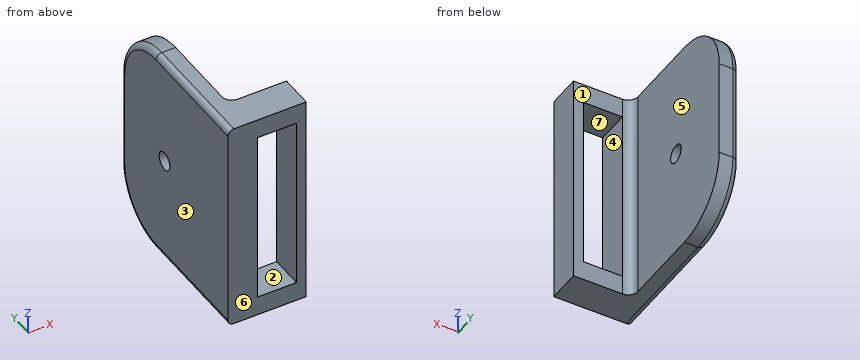
```python
from build123d import *

# Parameters (mm, degrees)
SKETCH1_W           = 40
SKETCH1_H           = 110
BOSS_EXTRUDE1_DEPTH = 17
SKETCH4_W           = 110
SKETCH4_H           = 75
BOSS_EXTRUDE2_DEPTH = 10
SKETCH5_W           = 20
SKETCH5_H           = 90
CUT_EXTRUDE1_DEPTH  = 17
SKETCH6_R           = 4.6
CUT_EXTRUDE2_DEPTH  = 10
FILLET1_R           = 30
FILLET2_R           = 3
FILLET3_R           = 5


with BuildPart() as part:
    # Sketch1 → Boss-Extrude1 (new body)
    with BuildSketch(Plane(origin=(0, 0, 0), x_dir=(1, 0, 0), z_dir=(0, 1, 0))):
        with Locations((20, 55)):
            Rectangle(SKETCH1_W, SKETCH1_H)
    extrude(amount=BOSS_EXTRUDE1_DEPTH)

    # Sketch4 → Boss-Extrude2 (add)
    with BuildSketch(Plane(origin=(0, 0, 0), x_dir=(0, 0, -1), z_dir=(1, 0, 0))):
        with Locations((55, 54.5)):
            Rectangle(SKETCH4_W, SKETCH4_H)
    extrude(amount=BOSS_EXTRUDE2_DEPTH)

    # Sketch5 → Cut-Extrude1 (cut)
    with BuildSketch(Plane(origin=(0, 17, 0), x_dir=(1, 0, 0), z_dir=(0, 1, 0))):
        with Locations((25, 55)):
            Rectangle(SKETCH5_W, SKETCH5_H)
    extrude(amount=-CUT_EXTRUDE1_DEPTH, mode=Mode.SUBTRACT)

    # Sketch6 → Cut-Extrude2 (cut)
    with BuildSketch(Plane(origin=(10, 0, 0), x_dir=(0, 0, -1), z_dir=(1, 0, 0))):
        with Locations((55, 54.7)):
            Circle(SKETCH6_R)
    extrude(amount=-CUT_EXTRUDE2_DEPTH, mode=Mode.SUBTRACT)

    # Fillet1
    fillet1_edges = [part.edges().sort_by_distance(p)[0] for p in [
        (5, 92, 0),
        (5, 92, -110),
    ]]
    fillet(fillet1_edges, radius=FILLET1_R)

    # Fillet2
    fillet2_edges = [part.edges().sort_by_distance(p)[0] for p in [
        (0, 31, 0),
        (0, 92, -55),
        (0, 31, -110),
        (0, 83.213203436, -101.213203436),
        (0, 83.213203436, -8.786796564),
    ]]
    fillet(fillet2_edges, radius=FILLET2_R)

    # Fillet3
    fillet3_edges = [part.edges().sort_by_distance(p)[0] for p in [
        (10, 17, -55),
    ]]
    fillet(fillet3_edges, radius=FILLET3_R - 0.0001)  # a hair under: the kernel refuses the full size


solid = part.part
```
Geometry: final body of the model. Coordinates: model frame, mm. Face numbers are marked on the shaded views. A direction names the side the tool comes from. Round coordinates to 2 decimals unless told otherwise and drop trailing zeros. Order: outer loops, then holes, each group sorted by start corner. A loop starts at its lowest first (then second) coordinate and runs counter-clockwise, first axis right, second up. Notation, with made-up numbers: (56.25, 27.25) -> (63.25, 27.25) arc R29 ccw to (63.25, 61.25) -> close; hole circle Ø11 at (-4, -24.75). An arc over 180 degrees is marked (long way). Use CSV: the item, a comma, the result in double quotes. Start each with the question number.
1) Section B-B (z = -55). State how many separate pieces and enclosed holes the cut face has, and give its area (3 significant figures).
2) First-contact query: pin 1 Ø4 at (y, z) = (41, -82.5) entering from +X; pin 2 Ø20 at (x, z) = (28, -42.5) entering from +Y. Flat tips, straight axial feed; report the tip coordinate or a pass-through.
3) Set-up query: the marked faces 1, 2 and 3. Return all of +Z, -Z, +X, -X, +Y, -Y with unobstructed straight access to the full face (end or side cutting, diameter ignored); none if empty.
4) Material intervals for line 1 along X through (y, z) = (15, -43); line 2 along Y through (x, z) = (7, -55); line 3 along X through (y, z) = (44, -85.5), sorted ascending. Write a range as from..to.
5) Section A-A (y = 54.7). Return the cut outline in (x, z).
6) Section C-C (x = 27). Return the cut outline in (y, z).
7) Section D-D (y = 15.5). Return the cut outline in (x, z).
8) Draft query along X for the marked faces 4, 5, 6 and 7. Return one class per face: +X half, -X half, draft (parallel to the pull), parting line (faces both ways), or undercut.
Returned:
1,separate pieces,"3"
1,enclosed holes,"0"
1,area,"1,000 mm²"
2,pin 1,"stops at x = 10"
2,pin 2,"stops at y = 17"
3,face 1,"+Z, -Z, +X, +Y"
3,face 2,"+Y, -Y"
3,face 3,"+Z, -Z, -X, +Y, -Y"
4,line 1,"x = 0..15, 35..40"
4,line 2,"y = 0..50.1, 59.3..92"
4,line 3,"x = 0..10"
5,outline,"(0, -107) arc R3 ccw to (3, -110) -> (10, -110) -> (10, -59.6) -> (0, -59.6) -> close; (0, -50.4) -> (10, -50.4) -> (10, 0) -> (3, 0) arc R3 ccw to (0, -3) -> close"
6,outline,"(0, -110) -> (17, -110) -> (17, -100) -> (0, -100) -> close; (0, -10) -> (17, -10) -> (17, 0) -> (0, 0) -> close"
7,outline,"(0, -107) arc R3 ccw to (3, -110) -> (40, -110) -> (40, 0) -> (3, 0) arc R3 ccw to (0, -3) -> close; hole (15, -100) -> (35, -100) -> (35, -10) -> (15, -10) -> close"
8,face 4,"undercut"
8,face 5,"+X half"
8,face 6,"draft"
8,face 7,"undercut"
